The model under review builds one solid part; all positions refer to its coordinate system, in mm. A direction names the side the tool comes from. Round coordinates to 2 decimals unless told otherwise and drop trailing zeros. Write each loop counter-clockwise with the first axis right and the second up, starting at its lowest first coordinate (ties: lowest second). Pieces come first, ordered by that corner, then holes. Notation, with made-up numbers: M 38.5,-29.5 L 53.5,-29.5 A26 ccw 53.5,-6.5 Z; hole C 29.25,3.5 d4. An arc over 180 degrees is marked long. Write item = value, one per line. Start each with the question number.
Item 1: To check wall thickness, follow line 1 along X through (y, z) = (-0.75, 0.25); line 2 along Z through (x, y) = (17.5, -15.25); line 3 along Z through (x, y) = (40.5, -12). State the ranges of each line that lie inside material, in increasing order.
Item 2: Take a section at C-C, the plane x = 57. Give the boundary of the cut face in (y, z), plus the area to 3 significant figures.
Item 3: For pin 1 Ø9.5 at (x, y) = (13, -9.5) entering from +Z, flat-tipped, find the tip position at first contact; note if it passes through.
Item 4: Take a section at B-B, the plane x = 76.5. Give the boundary of the cut face in (y, z).
Item 5: Take a section at A-A, the plane y = -2.75. Give the boundary of the cut face in (x, z), plus the area to 3 significant figures.
Item 6: Tool access review of faces 1 (the flat face through (50, -9, 0)), 2 (the flat face through (10, -9, 0.2)): name each direction out of +Z, -Z, +X, -X, +Y, -Y from which nothing blocks a thin tool from reaching the whole face with its end or side.
from build123d import *

# Parameters (mm, degrees)
F0_W     = 20.581514
F0_H     = 18.778749
F1_DEPTH = 0.2
F0_W_2   = 20.731736
F2_DEPTH = 0.3
F0_W_3   = 20.43128
F3_DEPTH = 0.4
F0_W_4   = 18.928978
F4_DEPTH = 0.5
F0_W_5   = 20.396158
F5_DEPTH = 0.6


with BuildPart() as f1:
    # F0 (on Top) → F1 (new body)
    with BuildSketch(Plane.XY):
        with Locations((10.290757, -9.389374)):
            Rectangle(F0_W, F0_H)
    extrude(amount=F1_DEPTH)

    # F0 (on Top) → F2 (join)
    with BuildSketch(Plane.XY):
        with Locations((30.947382, -9.389374)):
            Rectangle(F0_W_2, F0_H)
    extrude(amount=F2_DEPTH)

    # F0 (on Top) → F3 (join)
    with BuildSketch(Plane.XY):
        with Locations((51.52889, -9.389374)):
            Rectangle(F0_W_3, F0_H)
    extrude(amount=F3_DEPTH)

    # F0 (on Top) → F4 (join)
    with BuildSketch(Plane.XY):
        with Locations((71.209019, -9.389374)):
            Rectangle(F0_W_4, F0_H)
    extrude(amount=F4_DEPTH)

    # F0 (on Top) → F5 (join)
    with BuildSketch(Plane.XY):
        with Locations((90.871587, -9.389374)):
            Rectangle(F0_W_5, F0_H)
    extrude(amount=F5_DEPTH)


solid = f1.part
Response values:
q1.line_1 = 20.58 to 101.07
q1.line_2 = 0 to 0.2
q1.line_3 = 0 to 0.3
q2.outline = M -18.78,0 L 0,0 L 0,0.4 L -18.78,0.4 Z
q2.area = 7.51 mm2
q3.pin_1 = 0.2
q4.outline = M -18.78,0 L 0,0 L 0,0.5 L -18.78,0.5 Z
q5.outline = M 0,0 L 101.07,0 L 101.07,0.6 L 80.67,0.6 L 80.67,0.5 L 61.74,0.5 L 61.74,0.4 L 41.31,0.4 L 41.31,0.3 L 20.58,0.3 L 20.58,0.2 L 0,0.2 Z
q5.area = 40.2 mm2
q6.face_1 = -Z, +X, -X, +Y, -Y
q6.face_2 = +Z, -X, +Y, -Y
